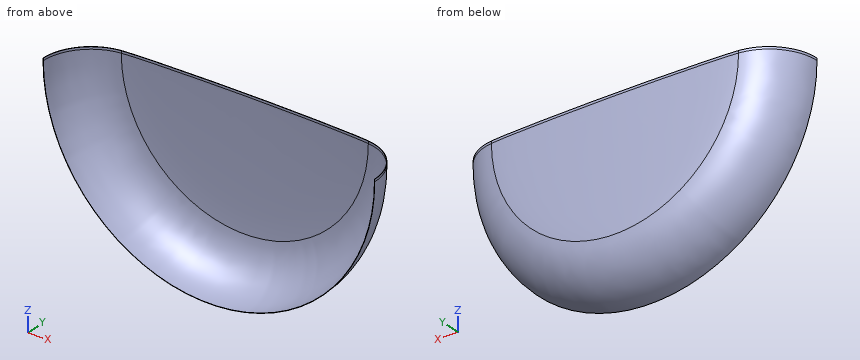
```python
from build123d import *

# Parameters (mm, degrees)
SURFACE_REVOLVE1_2_ANGLE = 180
SURFACE_EXTRUDE1_3_DEPTH = 15
THICKEN1_T2              = 2


with BuildPart() as body_1:
    # Surface-Revolve1: a surface, the sketch's curves turned about an axis by 180 degrees
    with BuildLine(Plane.XY, mode=Mode.PRIVATE) as surface_revolve1_2_path:
        ThreePointArc((0, 0), (79.571296782, 209.280495271), (278.084607626, 312.829432448))
        add(Edge.make_bspline(
            [(278.084607626, 312.829432448), (391.549286988, 326.218815687), (812.489449679, 335), (1095, 335)],
            knots=[0, 0, 0, 0, 1, 1, 1, 1], degree=3))
    surface_revolve1_2 = Shell.revolve(surface_revolve1_2_path.wire(), SURFACE_REVOLVE1_2_ANGLE, Axis((1095, 335, 0), (0, -1, 0)))
    # Surface-Extrude1: a surface, the sketch's curves swept straight by 15 mm
    with BuildLine(Plane.XY, mode=Mode.PRIVATE) as surface_extrude1_3_path:
        ThreePointArc((2190, 0), (2110.428703218, 209.280495271), (1911.915392374, 312.829432448))
        add(Edge.make_bspline(
            [(1911.915392374, 312.829432448), (1798.450713012, 326.218815687), (1377.510550321, 335), (1095, 335)],
            knots=[0, 0, 0, 0, 1, 1, 1, 1], degree=3))
        add(Edge.make_bspline(
            [(1095, 335), (812.489449679, 335), (391.549286988, 326.218815687), (278.084607626, 312.829432448)],
            knots=[0, 0, 0, 0, 1, 1, 1, 1], degree=3))
        ThreePointArc((278.084607626, 312.829432448), (79.571296782, 209.280495271), (0, 0))
    surface_extrude1_3 = Shell.extrude(surface_extrude1_3_path.wire(), (0 * SURFACE_EXTRUDE1_3_DEPTH, 0 * SURFACE_EXTRUDE1_3_DEPTH, 1 * SURFACE_EXTRUDE1_3_DEPTH))
    # Surface-Knit1: the surfaces knitted into one
    surface_knit1_1 = Shell(Face.sew_faces(surface_revolve1_2.faces() + surface_extrude1_3.faces())[0])
    add(Solid.thicken(surface_knit1_1, -THICKEN1_T2))


solid = body_1.part
```
Could you check a few things on this model? Use its own coordinates, in mm. Round coordinates to 2 decimals unless told otherwise and drop trailing zeros. Loops run counter-clockwise (first coordinate to the right, second up) from the corner with the lowest first, then second, coordinate; pieces in that order, holes last. Notation, with made-up numbers: M 67,-3 L 122,-3 A23 ccw 122,10 Z; hole C 70,43.5 d8. An arc over 180 degrees is marked long. Write item = value, one per line.
1. Will these pins go through, and if not, where does the flat tip stop? P1, Ø6, axis at y = 107.5, z = -135.5, coming from the -X side; P2, Ø4, axis at y = 251.5, z = -407.5, coming from the +X side; P3, Ø8, axis at y = 212.5, z = -557.5, coming from the -X side.
Results below:
P1 = 24.19
P2 = 1981.51
P3 = 241.55
2. I need wall thicknesses on probe 1 along X at (y, z) = (52, -479.5); probe 2 along X at (y, z) = (74.5, -195); probe 3 along Y at (x, z) = (2090, -168). Which ranges of each line are inside material? Lowest first, please.
Results below:
probe_1 = 113.12 to 115.38, 2074.62 to 2076.88
probe_2 = 24.49 to 26.59, 2163.41 to 2165.51
probe_3 = 216.21 to 219.11
3. I want a section at A-A, the plane y = 236.5. Write out the boundary of the cut face in (x, z).
Results below:
outline = M 103.92,0 A991.08 ccw 2086.08,0 L 2086.08,15 L 2083.07,15 L 2083.07,0 A988.07 cw 106.93,0 L 106.93,15 L 103.92,15 Z
